Input: part model. Units: mm. Frame: model coordinates. Face numbers are marked on the shaded views. A direction names the side the tool comes from. Give positions to 0.01 mm unless a question says otherwise; leave off trailing zeros. Loops run counter-clockwise (first coordinate to the right, second up) from the corner with the lowest first, then second, coordinate; pieces in that order, holes last.
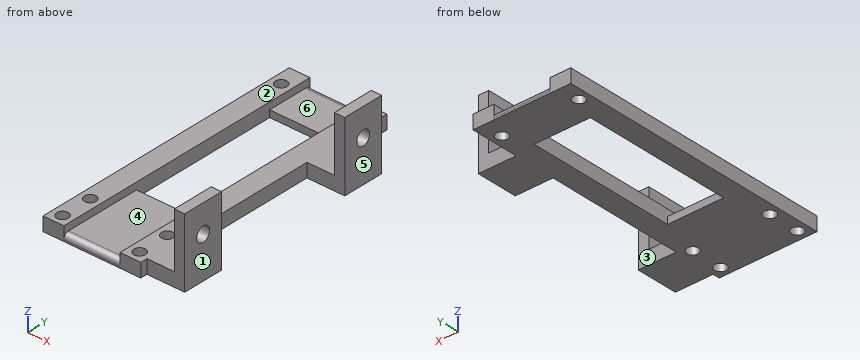
from build123d import *

# Parameters (mm, degrees)
SKETCH001_W     = 28.2
SKETCH001_H     = 80
PAD_DEPTH       = 4
SKETCH002_W     = 16.2
SKETCH002_H     = 80
POCKET_DEPTH    = 2
SKETCH003_W     = 16.2
SKETCH003_H     = 43.275
POCKET001_DEPTH = 2
SKETCH010_R     = 1.7
POCKET004_DEPTH = 4.001
SKETCH021_R     = 1.7
POCKET008_DEPTH = 4.001
FILLET_R        = 1.5
FILLET001_R     = 1.5
SKETCH025_W     = 12
SKETCH025_H     = 4
PAD009_DEPTH    = 10.9
SKETCH026_W     = 3
SKETCH026_H     = 12
PAD010_DEPTH    = 16
SKETCH027_R     = 2.1
POCKET010_DEPTH = 3.001


with BuildPart() as part:
    # Sketch001 → Pad (new body)
    with BuildSketch(Plane.XY):
        with Locations((0, -5.2375)):
            Rectangle(SKETCH001_W, SKETCH001_H)
    extrude(amount=PAD_DEPTH)

    # Sketch002 (on Face6 of Pad) → Pocket (cut)
    with BuildSketch(Plane.XY.offset(4)):
        with Locations((0, -5.2375)):
            Rectangle(SKETCH002_W, SKETCH002_H)
    extrude(amount=-POCKET_DEPTH, mode=Mode.SUBTRACT)

    # Sketch003 (on Face6 of Pocket) → Pocket001 (cut)
    with BuildSketch(Plane.XY.offset(2)):
        Rectangle(SKETCH003_W, SKETCH003_H)
    extrude(amount=-POCKET001_DEPTH, mode=Mode.SUBTRACT)

    # Sketch010 (on Face8 of Pocket001) → Pocket004 (cut, through all)
    with BuildSketch(Plane.XY.offset(4)):
        with Locations((-11.1, -42.2375)):
            Circle(SKETCH010_R)
        with Locations((-11.1, -33.2375)):
            Circle(SKETCH010_R)
        with Locations((11.1, -33.2375)):
            Circle(SKETCH010_R)
        with Locations((11.1, -42.2375)):
            Circle(SKETCH010_R)
    extrude(amount=-POCKET004_DEPTH, mode=Mode.SUBTRACT)

    # Sketch021 (on Face8 of Pocket004) → Pocket008 (cut, through all)
    with BuildSketch(Plane.XY.offset(4)):
        with Locations((-11.1, 28.7625)):
            Circle(SKETCH021_R)
        with Locations((11.1, 28.7625)):
            Circle(SKETCH021_R)
    extrude(amount=-POCKET008_DEPTH, mode=Mode.SUBTRACT)

    # Fillet
    fillet_edges = [part.edges().sort_by_distance(p)[0] for p in [
        (0, 34.7625, 2),
    ]]
    fillet(fillet_edges, radius=FILLET_R)

    # Fillet001
    fillet001_edges = [part.edges().sort_by_distance(p)[0] for p in [
        (0, -45.2375, 2),
    ]]
    fillet(fillet001_edges, radius=FILLET001_R)

    # Sketch025 (on Face15 of Fillet001) → Pad009 (join)
    with BuildSketch(Plane.YZ.offset(14.1)):
        with Locations((-37.2375, 2)):
            Rectangle(SKETCH025_W, SKETCH025_H)
        with Locations((14.7625, 2)):
            Rectangle(SKETCH025_W, SKETCH025_H)
    extrude(amount=PAD009_DEPTH)

    # Sketch026 (on Face28 of Pad009) → Pad010 (join)
    with BuildSketch(Plane.XY.offset(4)):
        with Locations((23.5, 14.7625)):
            Rectangle(SKETCH026_W, SKETCH026_H)
        with Locations((23.5, -37.2375)):
            Rectangle(SKETCH026_W, SKETCH026_H)
    extrude(amount=PAD010_DEPTH)

    # Sketch027 (on Face36 of Pad010) → Pocket010 (cut, through all)
    with BuildSketch(Plane(origin=(22, 0, 0), x_dir=(0, -1, 0), z_dir=(-1, 0, 0))):
        with Locations((-14.7625, 12)):
            Circle(SKETCH027_R)
        with Locations((37.2375, 12)):
            Circle(SKETCH027_R)
    extrude(amount=-POCKET010_DEPTH, mode=Mode.SUBTRACT)


solid = part.part
(1) Cut plane A-A (z = 12). Return the cut outline in (x, y).
Values follow:
outline: (22, -43.24) - (25, -43.24) - (25, -39.34) - (22, -39.34) - close; (22, -35.14) - (25, -35.14) - (25, -31.24) - (22, -31.24) - close; (22, 8.76) - (25, 8.76) - (25, 12.66) - (22, 12.66) - close; (22, 16.86) - (25, 16.86) - (25, 20.76) - (22, 20.76) - close
(2) Cut plane B-B (x = -11.1). Return the cut outline in (y, z).
Values follow:
outline: (-45.24, 0) - (-43.94, 0) - (-43.94, 4) - (-45.24, 4) - close; (-40.54, 0) - (-34.94, 0) - (-34.94, 4) - (-40.54, 4) - close; (-31.54, 0) - (27.06, 0) - (27.06, 4) - (-31.54, 4) - close; (30.46, 0) - (34.76, 0) - (34.76, 4) - (30.46, 4) - close
(3) Cut plane D-D (x = -6.5). Return the cut outline in (y, z).
Values follow:
outline: (-45.24, 0) - (-21.64, 0) - (-21.64, 2) - (-43.74, 2) arc R1.5 ccw to (-45.24, 0.5) - close; (21.64, 0) - (34.76, 0) - (34.76, 0.5) arc R1.5 ccw to (33.26, 2) - (21.64, 2) - close
(4) Cut plane C-C (y = 2.5). Return the cut outline in (x, z), and give its area (3 significant figures).
Values follow:
outline: (-14.1, 0) - (-8.1, 0) - (-8.1, 4) - (-14.1, 4) - close; (8.1, 0) - (14.1, 0) - (14.1, 4) - (8.1, 4) - close
area: 48.0 mm2
(5) Pin query (flat end, axial travel): pin 1 Ø2.5 at (y, z) = (-37.24, 12) entering from -X (3 decimals); pin 2 Ø5 at (x, y) = (0.5, -27.5) entering from +Z; pin 3 Ø5.5 at (x, z) = (19.5, 12.5) entering from -Y; pin 4 Ø12 at (x, y) = (-8.5, -18) entering from +Z. Return the tip coordinate at first contact, or that it passes through.
Values follow:
pin 1: passes through
pin 2: stops at z = 2
pin 3: stops at y = -43.24
pin 4: stops at z = 4
(6) Reachability of the marked faces 1 and 2 from +Z, -Z, +X, -X, +Y, -Y: full face, straight path, thin tool, end or side. Return the list, or none.
Values follow:
face 1: +Z, -Z, +X, +Y, -Y
face 2: +Z, -X, +Y, -Y
(7) Mould query, pull axis X, two halves, no side actions, for the marked faces 3, 4, 5 and 6. Classes: +X half, -X half, draft (parallel to the pull), parting line (faces both ways), or undercut.
Values follow:
face 3: draft
face 4: undercut
face 5: +X half
face 6: undercut
(8) Ray query, probe 1 along Y at (x, z) = (-11.1, 2.4); probe 2 along X at (y, z) = (-35, 3.25); probe 3 along Y at (x, z) = (23, 6.25). Return the intervals inside material, ascending.
Values follow:
probe 1: y = -45.24 to -43.94, -40.54 to -34.94, -31.54 to 27.06, 30.46 to 34.76
probe 2: x = -14.1 to -8.1, 8.1 to 25
probe 3: y = -43.24 to -31.24, 8.76 to 20.76
